```python
from build123d import *

# Parameters (mm, degrees)
CROQUIS1_W              = 26
CROQUIS1_H              = 12
SALIENTE_EXTRUIR1_DEPTH = 11
CROQUIS5_RX             = 5.5
CROQUIS5_RY             = 2
SALIENTE_EXTRUIR2_DEPTH = 26
CROQUIS6_RX             = 5.5
CROQUIS6_RY             = 2
SALIENTE_EXTRUIR3_DEPTH = 12
REVOLUCI_N2_ANGLE       = 90
CROQUIS9_R              = 3
CORTAR_EXTRUIR1_DEPTH   = 5
CROQUIS11_R             = 1.6
SALIENTE_EXTRUIR4_DEPTH = 14
CROQUIS12_R             = 2.1
CORTAR_EXTRUIR2_DEPTH   = 6


with BuildPart() as part:
    # Croquis1 → Saliente-Extruir1 (new body)
    with BuildSketch(Plane.XY):
        with Locations((-1.484877735, 3.639455782)):
            Rectangle(CROQUIS1_W, CROQUIS1_H)
    extrude(amount=SALIENTE_EXTRUIR1_DEPTH)

    # Croquis5 → Saliente-Extruir2 (add)
    with BuildSketch(Plane(origin=(11.515122265, 0, 0), x_dir=(0, 0, -1), z_dir=(1, 0, 0))):
        with Locations((-5.5, 9.639455782)):
            Ellipse(CROQUIS5_RX, CROQUIS5_RY)
    extrude(amount=-SALIENTE_EXTRUIR2_DEPTH)

    # Croquis6 → Saliente-Extruir3 (add)
    with BuildSketch(Plane.XZ.offset(2.360544218)):
        with Locations(Location((-14.484877735, 5.5), (0, 0, -90))):
            Ellipse(CROQUIS6_RX, CROQUIS6_RY)
    extrude(amount=-SALIENTE_EXTRUIR3_DEPTH)

    # Croquis8 → Revolución2 (revolve)
    with BuildSketch(Plane.ZY.offset(14.484877735)):
        with BuildLine():
            Line((0, 9.639455782), (11, 9.639455782))
            add(Edge.make_bspline(
                [(11, 9.639455782), (11, 11.639455782), (5.5, 11.639455782), (0, 11.639455782), (0, 9.639455782)],
                knots=[3.141592654, 3.141592654, 3.141592654, 4.71238898, 4.71238898, 6.283185307, 6.283185307, 6.283185307], degree=2, weights=[1, 0.707106781, 1, 0.707106781, 1]))
        make_face()
    revolve(axis=Axis((-14.484877735, 9.639455782, 0), (0, 0, 1)), revolution_arc=REVOLUCI_N2_ANGLE)

    # Croquis9 → Cortar-Extruir1 (cut)
    with BuildSketch(Plane(origin=(11.515122265, 0, 0), x_dir=(0, 0, -1), z_dir=(1, 0, 0))):
        with Locations((-5.5, 7.639455782)):
            Circle(CROQUIS9_R)
    extrude(amount=-CORTAR_EXTRUIR1_DEPTH, mode=Mode.SUBTRACT)

    # Croquis11 → Saliente-Extruir4 (add)
    with BuildSketch(Plane(origin=(6.515122265, 0, 0), x_dir=(0, 0, -1), z_dir=(1, 0, 0))):
        with Locations((-5.5, 7.639455782)):
            Circle(CROQUIS11_R)
    extrude(amount=SALIENTE_EXTRUIR4_DEPTH)

    # Croquis12 → Cortar-Extruir2 (cut)
    with BuildSketch(Plane.XZ.offset(2.360544218)):
        with Locations((1.515122265, 5.5)):
            Circle(CROQUIS12_R)
        with Locations((-6.484877735, 5.5)):
            Circle(CROQUIS12_R)
    extrude(amount=-CORTAR_EXTRUIR2_DEPTH, mode=Mode.SUBTRACT)


solid = part.part
```
Design review of the part built by this model. Coordinates are the model's own, in mm. A direction names the side the tool comes from. Coordinates: 2 decimals unless noted, no trailing zeros. Loops run counter-clockwise (first coordinate to the right, second up) from the corner with the lowest first, then second, coordinate; pieces in that order, holes last. Notation, with made-up numbers: (-27, 87) -> (-21, 87) arc R33 ccw to (-21, 126) -> close; hole circle Ø4 at (-19.75, 60.5). An arc over 180 degrees is marked (long way). Answer as a JSON object with one key per item and string values.
Q1. Tool access review of faces 4 (the cylindrical face through (9.05, 10.17, 3.89)), 5 (the flat face through (-2, 4, 0)), 6 (the cylindrical face through (-8.03, 0.6, 6.92)): name each direction out of +Z, -Z, +X, -X, +Y, -Y from which nothing blocks a thin tool from reaching the whole face with its end or side.
Answer block:
{"face 4": "+X", "face 5": "-Z, +X, -X, +Y, -Y", "face 6": "-Y"}
Q2. Take a section at A-A on y = 0.5. Give the number of separate pieces and of enclosed holes in the cut face, plus the area to 3 significant figures.
Answer block:
{"separate pieces": "1", "enclosed holes": "2", "area": "276 mm^2"}
Q3. To check wall thickness, follow L1, parallel to Y at x = 7.75, z = 5.5; L2, parallel to Z at x = 7.5, y = 5.5; L3, parallel to Z at x = 9.5, y = 6.25. State the ranges of each line that lie inside material, in increasing order.
Answer block:
{"L1": "y = -2.36 to 4.64, 6.04 to 9.24, 10.64 to 11.64", "L2": "z = 0 to 3.4, 7.6 to 11", "L3": "z = 0 to 2.84, 4.71 to 6.29, 8.16 to 11"}
Q4. Clearance check with flat-ended pins moving along their axes: pin 1 Ø3 at (x, z) = (16, 6) entering from -Y; pin 2 Ø4 at (y, z) = (0.5, 6) entering from +X; pin 3 Ø1.3 at (x, z) = (-6, 5) entering from -Y. State where each tip first meets the part, or that it passes through.
Answer block:
{"pin 1": "stops at y = 6.04", "pin 2": "stops at x = 11.52", "pin 3": "stops at y = 3.64"}
Q5. The part is to be moulded in two halves that separate along X. For faces 1 (the flat face through (-2, 4, 11)), 2 (the flat face through (-7, 3.639, 6)), 3 (the flat face through (11.515, 3, 6)), say which applies: +X half, -X half, draft (parallel to the pull), parting line (faces both ways), or undercut.
Answer block:
{"face 1": "draft", "face 2": "undercut", "face 3": "+X half"}
Q6. Take a section at B-B on x = 13. Give the boundary of the cut face in (y, z), plus the area to 3 significant figures.
Answer block:
{"outline": "circle Ø3.2 at (7.64, 5.5)", "area": "8.04 mm^2"}
